CAD build for the part. Positions are in the model's coordinates, mm. A direction names the side the tool comes from. Coordinates: 2 decimals unless noted, no trailing zeros. Loops run counter-clockwise (first coordinate to the right, second up) from the corner with the lowest first, then second, coordinate; pieces in that order, holes last.
1) Saw through at D-D, the plane x = -3.25. Write the cut outline in (y, z).
2) Saw through at C-C, the plane y = 0.1. Write the cut outline in (x, z).
3) Saw through at A-A, the plane x = 0. Write the cut outline in (y, z).
4) Which spindle directions (+Z, -Z, +X, -X, +Y, -Y) get a long thin tool onto all of the face, cutting with end or side? Do faces 4 (the flat face through (5, 0.4, 22.1)), 5 (the flat face through (0, -0.1, 17)), 6 (the cylindrical face through (0, 0.4, 31)), 7 (the flat face through (-5, 0.4, 21.5)). Say none if no direction does.
5) Pin check, flat tips, straight feed: pin 1 Ø0.6 at (y, z) = (0.5, 20) entering from -X; pin 2 Ø0.6 at (y, z) = (0.5, 34.5) entering from +X; pin 3 Ø3 at (x, z) = (3, 47) entering from -Y. Stop position of each tip, or through.
6) Saw through at B-B, the plane z = 47. Write the cut outline in (x, y).
7) Wall check: line 1 along Z through (x, y) = (0, 0.25); line 2 along Z through (x, y) = (-2.25, 0.3); line 3 along X through (y, z) = (0.8, 10). Give the ranges that are in metal, low to high.
8) Two-plate mould, pull along X, no slides. Class faces 1 (the flat face through (1, 0.4, 35)), 2 (the cylindrical face through (-0.1, 0.4, -5)), 3 (the flat face through (0, 1, 17)): +X half, -X half, draft (parallel to the pull), parting line (faces both ways), or undercut.
Solid Edge part; units mm, degrees
sketch "Sketch1" plane through (0, 0, 0) normal (0, -1, 0) x (1, 0, 0)
  circle A0 centre (0, 0) radius 1
  circle A1 centre (0, 47) radius 5
  line L0 (5, 43.6834) -> (5, 0)
  arc A2 (-5, 43.6834) -> (5, 43.6834) centre (0, 47) cw
  line L1 (-5, 0) -> (-5, 43.6834)
  arc A3 (5, 0) -> (-5, 0) centre (0, 0) cw
  line L2 (1, 32) -> (1, 38)
  arc A4 (-1, 32) -> (1, 32) centre (0, 32) ccw
  line L3 (-1, 38) -> (-1, 32)
  arc A5 (1, 38) -> (-1, 38) centre (0, 38) ccw
extrude "Extrusionsausprägung_1" add sketch "Sketch1" against normal blind 1 and the other way blind 0.1
Data:
1. outline: (-0.1, -3.8) - (1, -3.8) - (1, 43.2) - (-0.1, 43.2) - close; (-0.1, 50.8) - (1, 50.8) - (1, 52.04) - (-0.1, 52.04) - close
2. outline: (-5, 0) arc R5 ccw to (5, 0) - (5, 43.68) arc R6 ccw (long way) to (-5, 43.68) - close; hole circle Ø10 at (0, 47); hole circle Ø2 at (0, 0); hole (-1, 32) arc R1 ccw to (1, 32) - (1, 38) arc R1 ccw to (-1, 38) - close
3. outline: (-0.1, -5) - (1, -5) - (1, -1) - (-0.1, -1) - close; (-0.1, 1) - (1, 1) - (1, 31) - (-0.1, 31) - close; (-0.1, 39) - (1, 39) - (1, 42) - (-0.1, 42) - close; (-0.1, 52) - (1, 52) - (1, 53) - (-0.1, 53) - close
4. face 4: -Z, +X, +Y, -Y
4. face 5: +Z, -Z, +X, -X, -Y
4. face 6: +Y, -Y
4. face 7: -Z, -X, +Y, -Y
5. pin 1: stops at x = -5
5. pin 2: stops at x = 5
5. pin 3: passes through
6. outline: (-6, -0.1) - (-5, -0.1) - (-5, 1) - (-6, 1) - close; (5, -0.1) - (6, -0.1) - (6, 1) - (5, 1) - close
7. line 1: z = -5 to -1, 1 to 31, 39 to 42, 52 to 53
7. line 2: z = -4.47 to 42.53, 51.47 to 52.56
7. line 3: x = -5 to 5
8. face 1: undercut
8. face 2: parting line
8. face 3: draft
